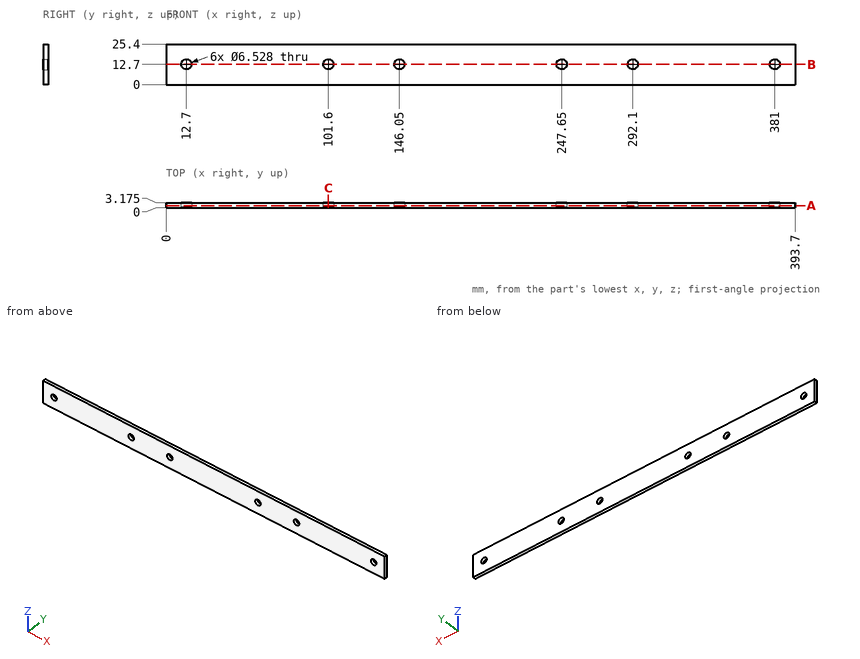
Drawing for the job (mm, zero at the part's lowest x, y, z). Give positions to 0.01 mm unless a question says otherwise; leave off trailing zeros. Write each loop counter-clockwise with the first axis right and the second up, starting at its lowest first coordinate (ties: lowest second). Pieces come first, ordered by that corner, then holes. Notation, with made-up numbers: M 9,42 L 22,42 A20 ccw 22,66 Z; hole C 35,14 d10. An arc over 180 degrees is marked long. Use CSV: the item, a comma, the result in double quotes.
Item 1: Drill centre lines: probe 1 along Z at (x, y) = (101.6, 1.75); probe 2 along Z at (x, y) = (246, 0.6). Where is each one in solid material? Low to high.
Taken from the geometry:
probe 1,"z = 0 to 9.44, 15.96 to 25.4"
probe 2,"z = 0 to 9.88, 15.52 to 25.4"
Item 2: Slice it at A-A on y = 1.3. Write the cut outline in (x, z).
Taken from the geometry:
outline,"M 0,0 L 393.7,0 L 393.7,25.4 L 0,25.4 Z; hole C 12.7,12.7 d6.53; hole C 101.6,12.7 d6.53; hole C 146.05,12.7 d6.53; hole C 247.65,12.7 d6.53; hole C 292.1,12.7 d6.53; hole C 381,12.7 d6.53"
Item 3: Slice it at C-C on x = 101.6. Write the cut outline in (y, z) (1 decimal), plus the area to 3 significant figures.
Taken from the geometry:
outline,"M 0,0 L 3.2,0 L 3.2,9.4 L 0,9.4 Z; M 0,16 L 3.2,16 L 3.2,25.4 L 0,25.4 Z"
area,"59.9 mm²"
Item 4: Slice it at B-B on z = 12.7. Write the cut outline in (x, y) (1 decimal), plus the area to 3 significant figures.
Taken from the geometry:
outline,"M 0,0 L 9.4,0 L 9.4,3.2 L 0,3.2 Z; M 16,0 L 98.3,0 L 98.3,3.2 L 16,3.2 Z; M 104.9,0 L 142.8,0 L 142.8,3.2 L 104.9,3.2 Z; M 149.3,0 L 244.4,0 L 244.4,3.2 L 149.3,3.2 Z; M 250.9,0 L 288.8,0 L 288.8,3.2 L 250.9,3.2 Z; M 295.4,0 L 377.7,0 L 377.7,3.2 L 295.4,3.2 Z; M 384.3,0 L 393.7,0 L 393.7,3.2 L 384.3,3.2 Z"
area,"1,130 mm²"
Item 5: Pin check, flat tip, straight feed: P1, Ø5, axis at x = 155.5, z = 2.5, coming from the -Y side. Stop position of the tip, or through.
Taken from the geometry:
P1,"stops at y = 0"
